The listing builds one solid part. Answer for the finished solid, in the listing's coordinates (mm). Face numbers are marked on the shaded views. Give positions to 0.01 mm unless a question says otherwise; leave off trailing zeros. Write each loop counter-clockwise with the first axis right and the second up, starting at its lowest first coordinate (ties: lowest second). Pieces come first, ordered by that corner, then holes. Notation, with made-up numbers: (-20, 16) -> (27, 16) arc R10 ccw to (27, 35) -> close; hole circle Ø8 at (71, 39.5). An arc over 180 degrees is marked (long way). Put each result on its own line as item: value. Start each with the question number.
1) A cutting plane is placed at B-B (y = 0). Write down the section's boundary in (x, z), then the cut area to 3 significant figures.
2) A cutting plane is placed at C-C (z = -165.1). Write down the section's boundary in (x, y), then the cut area to 3 significant figures.
3) A cutting plane is placed at A-A (z = 165.1). Write down the section's boundary in (x, y), then the cut area to 3 significant figures.
4) For a pull along Z with two mould halves and no side action, classify the marked faces 1, 2 and 3 as released by +Z, released by -Z, zero draft, split by the parting line, or undercut.
5) Find the intervals of material crossed by line 1 along Z through (x, y) = (19, 0.5); line 2 along Z through (x, y) = (5.75, 0); line 3 along Y through (x, z) = (11.25, -165.1), in increasing order. Write a range as from..to.
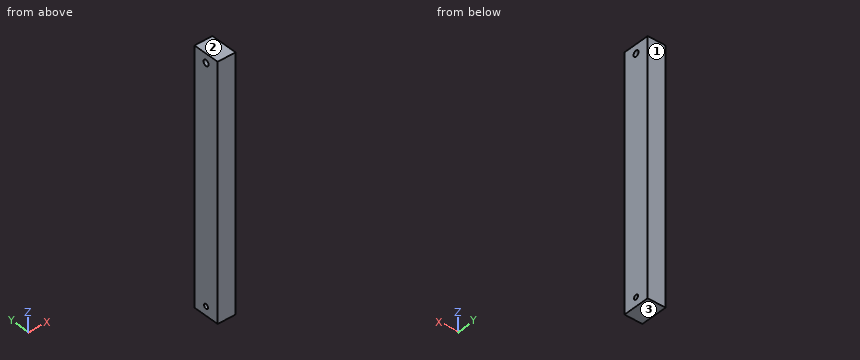
from build123d import *

# Parameters (mm, degrees)
F0_W     = 38.1
F0_H     = 355.6
F1_DEPTH = 25.4
F3_D     = 6.5278
F5_D     = 8.4328


with BuildPart() as f1:
    # F0 (on Right) → F1 (new body)
    with BuildSketch(Plane.YZ):
        Rectangle(F0_W, F0_H)
    extrude(amount=F1_DEPTH)

    # F3 (through all)
    with Locations(Plane.YZ.offset(25.4)):
        with Locations((0, -165.1)):
            Hole(F3_D / 2)

    # F5 (through all)
    with Locations(Plane.YZ.offset(25.4)):
        with Locations((0, 165.1)):
            Hole(F5_D / 2)


solid = f1.part
Reply:
1. outline: (0, -177.8) -> (25.4, -177.8) -> (25.4, -168.36) -> (0, -168.36) -> close; (0, -161.84) -> (25.4, -161.84) -> (25.4, 160.88) -> (0, 160.88) -> close; (0, 169.32) -> (25.4, 169.32) -> (25.4, 177.8) -> (0, 177.8) -> close
1. area: 8,650 mm2
2. outline: (0, -19.05) -> (25.4, -19.05) -> (25.4, -3.26) -> (0, -3.26) -> close; (0, 3.26) -> (25.4, 3.26) -> (25.4, 19.05) -> (0, 19.05) -> close
2. area: 802 mm2
3. outline: (0, -19.05) -> (25.4, -19.05) -> (25.4, -4.22) -> (0, -4.22) -> close; (0, 4.22) -> (25.4, 4.22) -> (25.4, 19.05) -> (0, 19.05) -> close
3. area: 754 mm2
4. face 1: zero draft
4. face 2: released by +Z
4. face 3: released by -Z
5. line 1: z = -177.8..-168.33, -161.87..160.91, 169.29..177.8
5. line 2: z = -177.8..-168.36, -161.84..160.88, 169.32..177.8
5. line 3: y = -19.05..-3.26, 3.26..19.05
